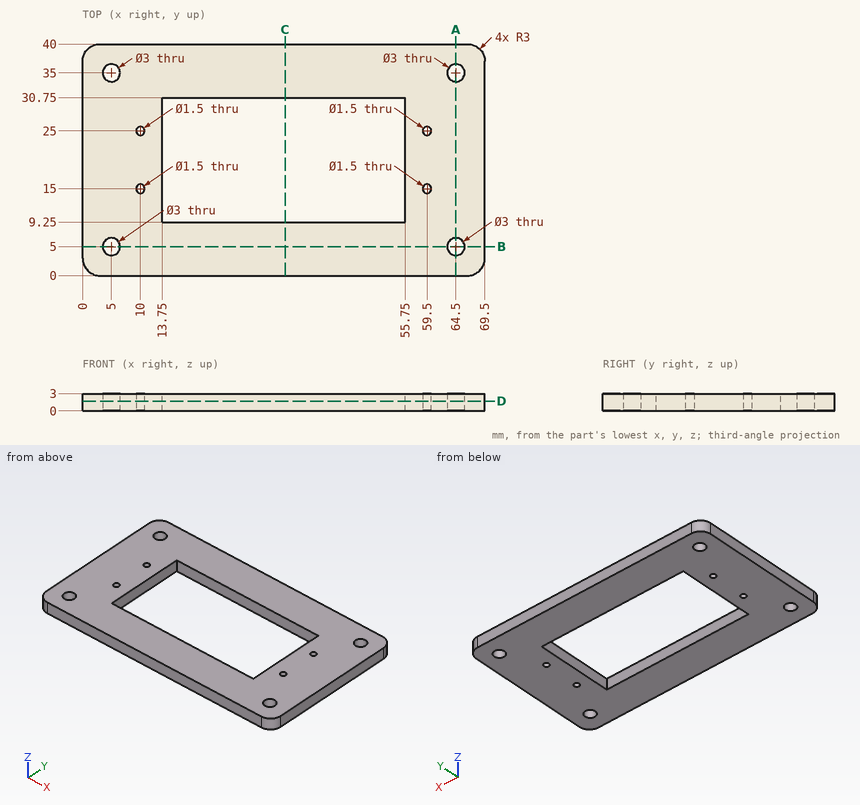
Study the drawing (mm; zero at the part's minimum x, y, z) and answer. Give positions to 0.01 mm unless a question says otherwise; leave off trailing zeros. Write each loop counter-clockwise with the first axis right and the second up, starting at its lowest first coordinate (ties: lowest second). Pieces come first, ordered by that corner, then holes. Notation, with made-up numbers: (57, 42) -> (87, 42) arc R12 ccw to (87, 51) -> close; hole circle Ø10 at (78, 80). An arc over 180 degrees is marked (long way). Write item = value, one per line. Start each with the question number.
1) The part is cut by section D-D, the plane z = 1.7. Count the separate pieces of the cut face and the enclosed holes in it, and give its area (3 significant figures).
2) The part is cut by section B-B, the plane y = 5. Determine the outline of the cut face in (x, z), and give its area (4 significant figures).
3) The part is cut by section C-C, the plane x = 35. Determine the outline of the cut face in (y, z), and give its area (3 significant figures).
4) Straight lines are drawn through the part: line 1 along Y through (x, z) = (10, 1.25); line 2 along X through (y, z) = (19, 0.35); line 3 along Y through (x, z) = (10.5, 1.85). For each, find the intervals that lie inside material, in ascending order.
5) The part is cut by section A-A, the plane x = 64.5. Determine the outline of the cut face in (y, z), and give its area (3 significant figures).
Solutions:
q1.separate_pieces = 1
q1.enclosed_holes = 9
q1.area = 1,830 mm²
q2.outline = (0, 0) -> (3.5, 0) -> (3.5, 3) -> (0, 3) -> close; (6.5, 0) -> (63, 0) -> (63, 3) -> (6.5, 3) -> close; (66, 0) -> (69.5, 0) -> (69.5, 3) -> (66, 3) -> close
q2.area = 190.5 mm²
q3.outline = (0, 0) -> (9.25, 0) -> (9.25, 3) -> (0, 3) -> close; (30.75, 0) -> (40, 0) -> (40, 3) -> (30.75, 3) -> close
q3.area = 55.5 mm²
q4.line_1 = 0 to 14.25, 15.75 to 24.25, 25.75 to 40
q4.line_2 = 0 to 13.75, 55.75 to 69.5
q4.line_3 = 0 to 14.44, 15.56 to 24.44, 25.56 to 40
q5.outline = (0, 0) -> (3.5, 0) -> (3.5, 3) -> (0, 3) -> close; (6.5, 0) -> (33.5, 0) -> (33.5, 3) -> (6.5, 3) -> close; (36.5, 0) -> (40, 0) -> (40, 3) -> (36.5, 3) -> close
q5.area = 102 mm²
